Work out the finished part from the listing and answer in its coordinate system (mm). Coordinates: 2 decimals unless noted, no trailing zeros. Write each loop counter-clockwise with the first axis right and the second up, starting at its lowest first coordinate (ties: lowest second). Pieces come first, ordered by that corner, then holes. Notation, with made-up numbers: (18, 20.25) -> (22, 20.25) arc R13 ccw to (22, 45.25) -> close; hole circle Ø8 at (43.5, 88). An arc over 180 degrees is marked (long way). Write each question's results on one line, items separated by ' | '. Start each with the question number.
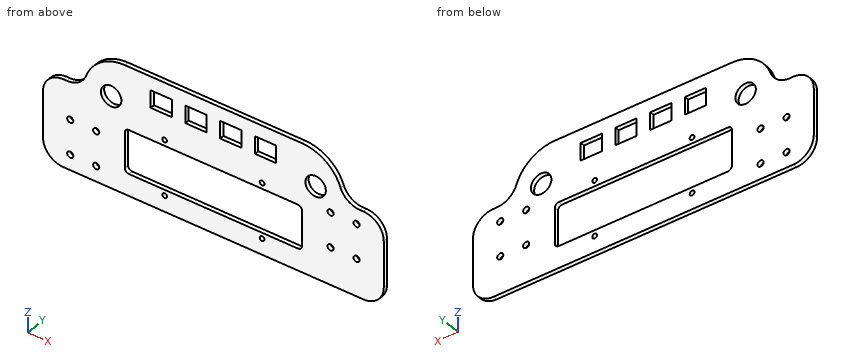
from build123d import *

# Parameters (mm, degrees)
SKETCH3_W            = 130
SKETCH3_H            = 32
SKETCH3_R            = 1.75
BOSS_EXTRUDE1_DEPTH  = 3.175
M4_CLEARANCE_HOLE1_D = 4.5
FILLET1_R            = 15
SKETCH6_W            = 15.5
SKETCH6_H            = 12.8
CUT_EXTRUDE1_DEPTH   = 140.56747696
SKETCH7_R            = 7.5
CUT_EXTRUDE2_DEPTH   = 140.56747696
FILLET2_R            = 3


with BuildPart() as part:
    # Sketch3 → Boss-Extrude1 (new body)
    with BuildSketch(Plane(origin=(0, 0, 0), x_dir=(1, 0, 0), z_dir=(0, 1, 0))):
        with BuildLine():
            Line((-125, 32), (-125, -32))
            Line((-125, -32), (-95, -32))
            ThreePointArc((-95, -32), (-86.213203436, -53.213203436), (-65, -62))
            Line((-65, -62), (65, -62))
            ThreePointArc((65, -62), (86.213203436, -53.213203436), (95, -32))
            Line((95, -32), (125, -32))
            Line((125, -32), (125, 32))
            Line((125, 32), (-125, 32))
        make_face()
        Rectangle(SKETCH3_W, SKETCH3_H, mode=Mode.SUBTRACT)
        with Locations(Location((-35.75, 20.25, 0), (0, 0, 270))):
            Circle(SKETCH3_R, mode=Mode.SUBTRACT)
        with Locations(Location((35.75, 20.25, 0), (0, 0, 270))):
            Circle(SKETCH3_R, mode=Mode.SUBTRACT)
        with Locations(Location((-35.75, -20.25, 0), (0, 0, 270))):
            Circle(SKETCH3_R, mode=Mode.SUBTRACT)
        with Locations(Location((35.75, -20.25, 0), (0, 0, 270))):
            Circle(SKETCH3_R, mode=Mode.SUBTRACT)
    extrude(amount=BOSS_EXTRUDE1_DEPTH)

    # M4 Clearance Hole1 (through all)
    with Locations(Plane(origin=(0, 3.175, 0), x_dir=(1, 0, 0), z_dir=(0, 1, 0))):
        with Locations((-105.025, 20.7), (-85.975, 20.7), (-105.025, -4.7), (-85.975, -4.7), (85.975, 4.7), (105.025, 4.7), (105.025, -20.7), (85.975, -20.7)):
            Hole(M4_CLEARANCE_HOLE1_D / 2)

    # Fillet1
    fillet1_edges = [part.edges().sort_by_distance(p)[0] for p in [
        (-125, 1.5875, 32),
        (-125, 1.5875, -32),
        (125, 1.5875, -32),
        (125, 1.5875, 32),
        (95, 1.5875, 32),
        (-95, 1.5875, 32),
    ]]
    fillet(fillet1_edges, radius=FILLET1_R)

    # Sketch6 → Cut-Extrude1 (cut, through all)
    with BuildSketch(Plane(origin=(0, 3.175, 0), x_dir=(1, 0, 0), z_dir=(0, 1, 0))):
        with Locations((-38.25, -45.6)):
            Rectangle(SKETCH6_W, SKETCH6_H)
        with Locations((-12.75, -45.6)):
            Rectangle(SKETCH6_W, SKETCH6_H)
    cut_extrude1 = extrude(amount=-CUT_EXTRUDE1_DEPTH, mode=Mode.SUBTRACT)

    # Sketch7 → Cut-Extrude2 (cut, through all)
    with BuildSketch(Plane(origin=(0, 3.175, 0), x_dir=(1, 0, 0), z_dir=(0, 1, 0))):
        with Locations(Location((-75, -35, 0), (0, 0, 270))):
            Circle(SKETCH7_R)
    cut_extrude2 = extrude(amount=-CUT_EXTRUDE2_DEPTH, mode=Mode.SUBTRACT)

    # Mirror1: Cut-Extrude1, Cut-Extrude2 across plane
    add(cut_extrude1.mirror(Plane(origin=(0, 0, 0), x_dir=(0, 0, 1), z_dir=(1, 0, 0))), mode=Mode.SUBTRACT)
    add(cut_extrude2.mirror(Plane(origin=(0, 0, 0), x_dir=(0, 0, 1), z_dir=(1, 0, 0))), mode=Mode.SUBTRACT)

    # Fillet2
    fillet2_edges = [part.edges().sort_by_distance(p)[0] for p in [
        (65, 1.5875, 16),
        (65, 1.5875, -16),
        (-65, 1.5875, -16),
        (-65, 1.5875, 16),
    ]]
    fillet(fillet2_edges, radius=FILLET2_R)


solid = part.part
1. Find the intervals of material crossed by L1, parallel to Z at x = -13.5, y = 0.7; L2, parallel to Z at x = 3, y = 0.25; L3, parallel to X at y = 0.6, z = 29, in increasing order.
2. Find section B-B on x = -70.5. Give the vertices of the cut face in (y, z) (3 decimals).
3. Find section A-A on z = 4.7. Give the vertices of the cut face in (x, y) (3 decimals).
4. Given pin 1 Ø0.8 at (x, y) = (-108, 1.5) entering from +Z; pin 2 Ø1 at (x, y) = (73, 2) entering from +Z, each flat-ended and moving along its own axis, determine where each tip first touches the part or whether it passes through.
5. Find section D-D on z = 35. Give the vertices of the cut face in (x, y) (3 decimals).
6. Find section C-C on y = 1. Give the number of separate pieces and of enclosed holes in the cut face, and give its area (3 significant figures).
Ans:
1) L1: z = -32 to -16, 16 to 39.2, 52 to 62 | L2: z = -32 to -16, 16 to 62 | L3: x = -119 to -79.5, -70.5 to 70.5, 79.5 to 119
2) outline: (0, -32) -> (3.175, -32) -> (3.175, 29) -> (0, 29) -> close; (0, 41) -> (3.175, 41) -> (3.175, 61.492) -> (0, 61.492) -> close
3) outline: (-125, 0) -> (-107.275, 0) -> (-107.275, 3.175) -> (-125, 3.175) -> close; (-102.775, 0) -> (-88.225, 0) -> (-88.225, 3.175) -> (-102.775, 3.175) -> close; (-83.725, 0) -> (-65, 0) -> (-65, 3.175) -> (-83.725, 3.175) -> close; (65, 0) -> (125, 0) -> (125, 3.175) -> (65, 3.175) -> close
4) pin 1: stops at z = 32 | pin 2: stops at z = 61.05
5) outline: (-98.426, 0) -> (-82.5, 0) -> (-82.5, 3.175) -> (-98.426, 3.175) -> close; (-67.5, 0) -> (67.5, 0) -> (67.5, 3.175) -> (-67.5, 3.175) -> close; (82.5, 0) -> (98.426, 0) -> (98.426, 3.175) -> (82.5, 3.175) -> close
6) separate pieces: 1 | enclosed holes: 19 | area: 15,700 mm²
